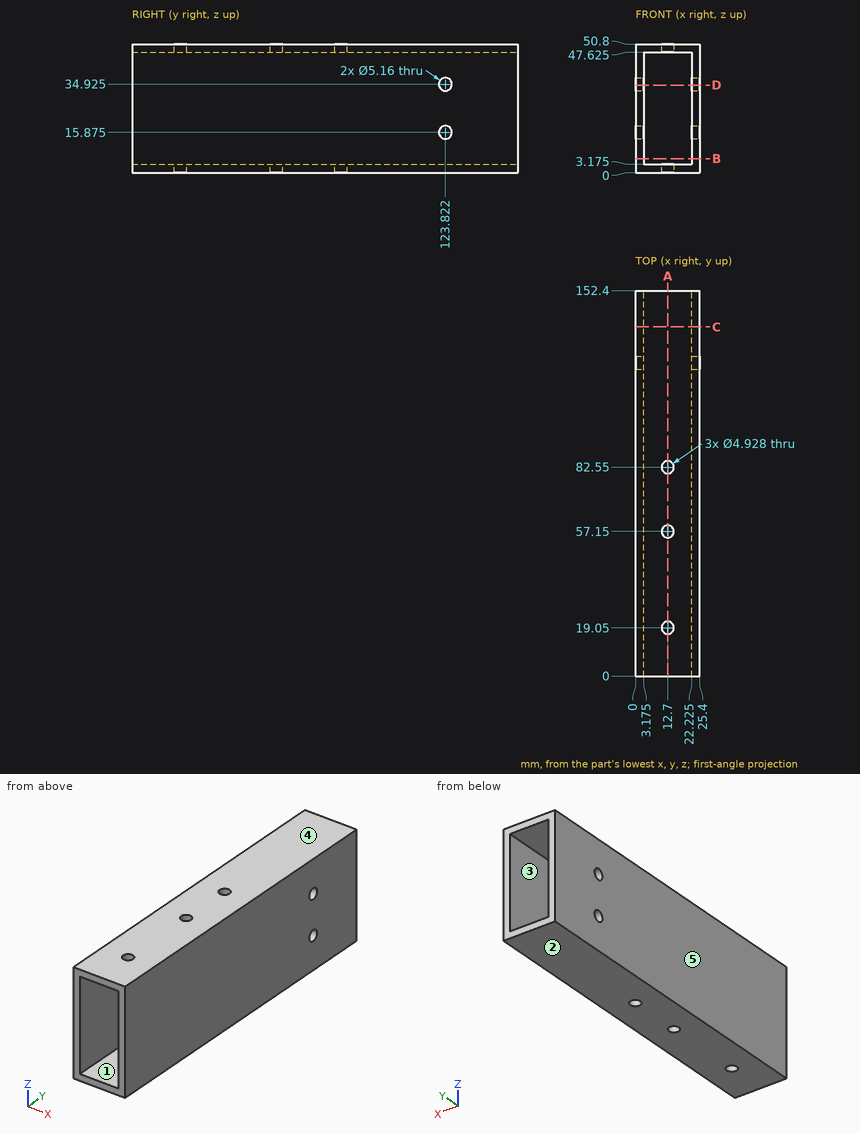
The figure shows three views and two pictorial views of one solid part (mm, origin at its lowest corner). Answer the questions. A direction names the side the tool comes from. Round coordinates to 2 decimals unless told otherwise and drop trailing zeros. Order: outer loops, then holes, each group sorted by start corner. A loop starts at its lowest first (then second) coordinate and runs counter-clockwise, first axis right, second up. Notation, with made-up numbers: (-34, -16) - (7, -16) arc R23 cw to (7, 1) - close; hole circle Ø3 at (66.5, 18.5). An arc over 180 degrees is marked (long way). Write item = value, one per line. Start each with the question number.
1) For a pull along Z with two mould halves and no side action, classify the marked faces 3, 4 and 5 as released by +Z, released by -Z, zero draft, split by the parting line, or undercut.
2) Section A-A, the plane x = 12.7 is taken. Count the separate pieces of the cut face and the enclosed holes in it.
3) Section C-C, the plane y = 138 is taken. Write down the section's boundary in (x, z) (1 decimal).
4) Straight lines are drawn through the part: L1, parallel to Y at x = 12.7, z = 1.6; L2, parallel to X at y = 61.5, z = 5 (1 decimal); L3, parallel to Z at x = 9.5, y = 34 (1 decimal). For each, find the intervals that lie inside material, in ascending order.
5) For the marked faces 1 and 2, determine the directions among +Z, -Z, +X, -X, +Y, -Y from which every point of the face is accessible in a straight line to the end or side of a thin tool.
6) Section B-B, the plane z = 5.5 is taken. Write down the section's boundary in (x, y) (1 decimal).
7) Given pin 1 (4.5 mm diameter, centred on y = 123.82, z = 34.92, fed in from +X), flat-ended and moving along its own axis, determine where the tip first touches the part or whether it passes through.
8) Section D-D, the plane z = 34.5 is taken. Write down the section's boundary in (x, y) (1 decimal).
Results list:
q1.face_3 = undercut
q1.face_4 = released by +Z
q1.face_5 = zero draft
q2.separate_pieces = 8
q2.enclosed_holes = 0
q3.outline = (0, 0) - (25.4, 0) - (25.4, 50.8) - (0, 50.8) - close; hole (3.2, 3.2) - (22.2, 3.2) - (22.2, 47.6) - (3.2, 47.6) - close
q4.L1 = 0 to 16.59, 21.51 to 54.69, 59.61 to 80.09, 85.01 to 152.4
q4.L2 = 0 to 3.2, 22.2 to 25.4
q4.L3 = 0 to 3.2, 47.6 to 50.8
q5.face_1 = +Y, -Y
q5.face_2 = -Z, +X, -X, +Y, -Y
q6.outline = (0, 0) - (3.2, 0) - (3.2, 152.4) - (0, 152.4) - close; (22.2, 0) - (25.4, 0) - (25.4, 152.4) - (22.2, 152.4) - close
q7.pin_1 = through
q8.outline = (0, 0) - (3.2, 0) - (3.2, 121.3) - (0, 121.3) - close; (0, 126.4) - (3.2, 126.4) - (3.2, 152.4) - (0, 152.4) - close; (22.2, 0) - (25.4, 0) - (25.4, 121.3) - (22.2, 121.3) - close; (22.2, 126.4) - (25.4, 126.4) - (25.4, 152.4) - (22.2, 152.4) - close
